Part model, mm, in its own coordinate system. Face numbers are marked on the shaded views. A direction names the side the tool comes from. Coordinates: 2 decimals unless noted, no trailing zeros. Write each loop counter-clockwise with the first axis right and the second up, starting at its lowest first coordinate (ties: lowest second). Pieces come first, ordered by that corner, then holes. Notation, with made-up numbers: (-0.5, 24.25) -> (58.5, 24.25) arc R27 cw to (58.5, 47.25) -> close; hole circle Ø11 at (1, 65.5). An arc over 180 degrees is marked (long way). Write item = value, one per line. Start each with the question number.
Q1. Pull direction Z, two halves, no side cores. Call the marked faces 3, 4 and 5: released by +Z, released by -Z, zero draft, split by the parting line, or undercut.
Q2. Band-saw the part on D-D, the plane x = 11. List the corners of the cut face in (y, z), plus the area to 3 significant figures.
Q3. Band-saw the part on A-A, the plane y = 7. List the corners of the cut face in (x, z).
Q4. Band-saw the part on C-C, the plane z = 4.5. List the corners of the cut face in (x, y).
Q5. Tool access for the marked faces 1 and 2: list every direction of +Z, -Z, +X, -X, +Y, -Y with a clear straight run to the whole face (end or side of a thin tool).
Q6. Band-saw the part on B-B, the plane x = 6.75. List the corners of the cut face in (y, z).
Q7. Probe line 1 (Y direction, x = 5.75, z = 22); line 2 (X direction, y = 8, z = 18.5); line 3 (Z direction, x = 1.5, y = 1.5). List the from-to ranges inside material, lowest first.
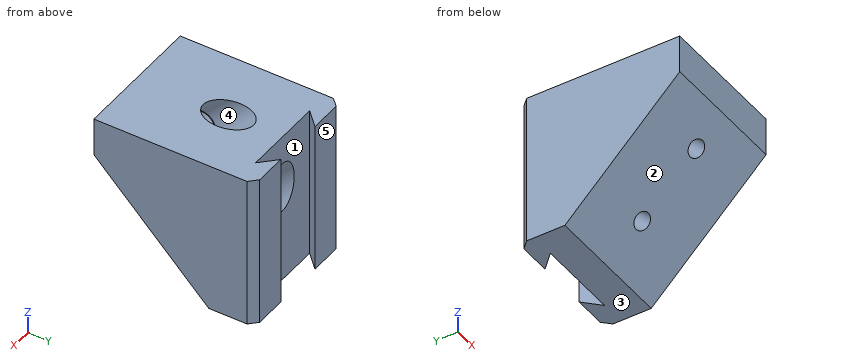
from build123d import *

# Parameters (mm, degrees)
BOSS_EXTRUDE1_DEPTH                                  = 30
BOSS_EXTRUDE2_DEPTH                                  = 26
CUT_EXTRUDE1_REACH                                   = 41.613
SKETCH8_R                                            = 3.5
CSK_FOR_M3_HEX_SOCKET_COUNTERSUNK_CAP_SC_D           = 3.4
CSK_FOR_M3_HEX_SOCKET_COUNTERSUNK_CAP_SC_CSINK_D     = 6.72
CSK_FOR_M3_HEX_SOCKET_COUNTERSUNK_CAP_SC_CSINK_ANGLE = 90


with BuildPart() as part:
    # Sketch2 → Boss-Extrude1 (new body)
    with BuildSketch(Plane.XY):
        Polygon((-13, 0), (13, 0), (13, 7.5), (11.5, 9), (5.15, 9), (8.15, 6), (-8.15, 6), (-5.15, 9), (-11.5, 9), (-13, 7.5), align=None)
    extrude(amount=BOSS_EXTRUDE1_DEPTH)

    # Sketch3 → Boss-Extrude2 (add)
    with BuildSketch(Plane(origin=(13, 0, 0), x_dir=(0, 0, -1), z_dir=(1, 0, 0))):
        Polygon((-30, 0), (-30, -22.5), (-22.5, -22.5), (0, 0), align=None)
    extrude(amount=-BOSS_EXTRUDE2_DEPTH)

    # Sketch8 → Cut-Extrude1 (cut, up to next)
    with BuildSketch(Plane(origin=(0, 7.071067812, 7.071067812), x_dir=(1, 0, 0), z_dir=(0, 0.7071067811865462, 0.7071067811865489)), mode=Mode.PRIVATE) as cut_extrude1_sk1:
        with Locations(Location((0, -9.470562748, 0), (0, 0, 90))):
            Circle(SKETCH8_R)
    cut_extrude1_tool1 = extrude(cut_extrude1_sk1.sketch, amount=CUT_EXTRUDE1_REACH, mode=Mode.PRIVATE) & part.part
    # Sketch8 → Cut-Extrude1 (cut, up to next)
    with BuildSketch(Plane(origin=(0, 7.071067812, 7.071067812), x_dir=(1, 0, 0), z_dir=(0, 0.7071067811865462, 0.7071067811865489)), mode=Mode.PRIVATE) as cut_extrude1_sk2:
        with Locations(Location((0, -24.470562748, 0), (0, 0, 270))):
            Circle(SKETCH8_R)
    cut_extrude1_tool2 = extrude(cut_extrude1_sk2.sketch, amount=CUT_EXTRUDE1_REACH, mode=Mode.PRIVATE) & part.part
    add(cut_extrude1_tool1.solids().sort_by_distance((0, 0.374369, 13.767767))[0], mode=Mode.SUBTRACT)
    add(cut_extrude1_tool2.solids().sort_by_distance((0, -10.232233, 24.374369))[0], mode=Mode.SUBTRACT)

    # CSK for M3 Hex Socket Countersunk Cap Screw3 (through all)
    with Locations(Plane(origin=(0, 7.071067812, 7.071067812), x_dir=(1, 0, 0), z_dir=(0, 0.7071067811865462, 0.7071067811865489))):
        with Locations((0, -9.470562748), (0, -24.470562748)):
            CounterSinkHole(CSK_FOR_M3_HEX_SOCKET_COUNTERSUNK_CAP_SC_D / 2, CSK_FOR_M3_HEX_SOCKET_COUNTERSUNK_CAP_SC_CSINK_D / 2, counter_sink_angle=CSK_FOR_M3_HEX_SOCKET_COUNTERSUNK_CAP_SC_CSINK_ANGLE)


solid = part.part
Ans:
q1.face_3 = released by -Z
q1.face_4 = undercut
q1.face_5 = zero draft
q2.outline = (-22.5, 22.5) -> (0, 0) -> (9, 0) -> (9, 30) -> (-22.5, 30) -> close
q2.area = 692 mm2
q3.outline = (-13, 0) -> (-7.15, 0) -> (-7.15, 30) -> (-13, 30) -> close; (7.15, 0) -> (13, 0) -> (13, 30) -> (7.15, 30) -> close
q4.outline = (-13, -4.5) -> (13, -4.5) -> (13, 7.5) -> (11.5, 9) -> (5.15, 9) -> (8.15, 6) -> (-8.15, 6) -> (-5.15, 9) -> (-11.5, 9) -> (-13, 7.5) -> close
q5.face_1 = +Z, -Z
q5.face_2 = -Z, +X, -X, -Y
q6.outline = (-22.5, 22.5) -> (0, 0) -> (6, 0) -> (6, 30) -> (-22.5, 30) -> close; (7.4, 0) -> (9, 0) -> (9, 30) -> (7.4, 30) -> close
q7.line_1 = -22 to 6, 8.4 to 9
q7.line_2 = -12.5 to -6.15, 6.15 to 12.5
q7.line_3 = 0 to 11.71, 19.37 to 30
